```python
from build123d import *

# Parameters (mm, degrees)
SKETCH1_W                    = 120
SKETCH1_H                    = 72
BOSS_EXTRUDE1_DEPTH          = 10
FILLET1_R                    = 10
M12_TAPPED_HOLE1_D           = 10.2
M12_TAPPED_HOLE1_CSINK_D     = 12.05
M12_TAPPED_HOLE1_CSINK_ANGLE = 90
BOSS_EXTRUDE2_START          = 10
SKETCH4_W                    = 50
SKETCH4_H                    = 72
BOSS_EXTRUDE2_DEPTH          = 3
CUT_EXTRUDE1_DEPTH           = 72.168813395
CUT_EXTRUDE1_DEPTH_BACK      = 72.168813395


with BuildPart() as part:
    # Sketch1 → Boss-Extrude1 (new body)
    with BuildSketch(Plane(origin=(0, 0, 0), x_dir=(1, 0, 0), z_dir=(0, 1, 0))):
        Rectangle(SKETCH1_W, SKETCH1_H)
    extrude(amount=BOSS_EXTRUDE1_DEPTH)

    # Fillet1
    fillet1_edges = [part.edges().sort_by_distance(p)[0] for p in [
        (60, 5, 36),
        (-60, 5, 36),
        (-60, 5, -36),
        (60, 5, -36),
    ]]
    fillet(fillet1_edges, radius=FILLET1_R)

    # M12 Tapped Hole1 (through all)
    with Locations(Plane.XZ):
        with Locations((-50, -26), (50, -26), (50, 26), (-50, 26)):
            CounterSinkHole(M12_TAPPED_HOLE1_D / 2, M12_TAPPED_HOLE1_CSINK_D / 2, counter_sink_angle=M12_TAPPED_HOLE1_CSINK_ANGLE)

    # Sketch4 → Boss-Extrude2 (add)
    with BuildSketch(Plane(origin=(0, 0, 0), x_dir=(1, 0, 0), z_dir=(0, 1, 0)).offset(BOSS_EXTRUDE2_START)):
        Rectangle(SKETCH4_W, SKETCH4_H)
    extrude(amount=BOSS_EXTRUDE2_DEPTH)

    # Sketch5 → Cut-Extrude1 (cut, two sides: drawn at the far end of the back side and taken through both)
    with BuildSketch(Plane.XY.offset(-CUT_EXTRUDE1_DEPTH_BACK)):
        Polygon((-28, 0), (-25, 3), (25, 3), (28, 0), align=None)
    extrude(amount=CUT_EXTRUDE1_DEPTH + CUT_EXTRUDE1_DEPTH_BACK, mode=Mode.SUBTRACT)


solid = part.part
```
The listing builds one solid part. Answer for the finished solid, in the listing's coordinates (mm). A direction names the side the tool comes from. Coordinates: 2 decimals unless noted, no trailing zeros. Loops run counter-clockwise (first coordinate to the right, second up) from the corner with the lowest first, then second, coordinate; pieces in that order, holes last. Notation, with made-up numbers: M 46.25,79.25 L 66.25,79.25 A24 ccw 66.25,103.25 Z; hole C -17,7.5 d7. An arc over 180 degrees is marked long. Answer as a JSON object with one key per item and string values. Group by question number.
Item 1: Determine the mould class of faces 1 (the face through (0, 13, -1)), 2 (the face through (-27, 1, -1)), 3 (the face through (-57.15, 5.07, 32.99)) for opening direction X: +X half, -X half, draft (parallel to the pull), parting line (faces both ways), or undercut.
Item 2: Consider L1, parallel to X at y = 5.25, z = 26; L2, parallel to Z at x = 50, y = 4.75; L3, parallel to X at y = 6, z = -28.5. Determine where each line is inside the solid, lowest interval first.
Item 3: Which of the six approach directions +Z, -Z, +X, -X, +Y, -Y give full straight-line access (tool end or side, diameter ignored) to faces 4 (the face through (-25, 11, 1)), 5 (the face through (42, 10, -1)), 6 (the face through (26, 2, -1)), 7 (the face through (54.05, 5.53, -29.1))?
Item 4: Section B-B (x = 17.5) is taken. Write down the section's boundary in (y, z), and give its area (3 significant figures).
Item 5: Section C-C (y = 11.5) is taken. Write down the section's boundary in (x, z), and give its area (3 significant figures).
Item 6: Each of these flat-tipped pins is pushed along its axis until it touches: P1, Ø6, axis at x = -50, z = 26, coming from the -Y side (3 decimals); P2, Ø11.5, axis at x = -50, z = -26, coming from the +Y side; P3, Ø3, axis at x = -37, y = 10.5, coming from the +Z side; P4, Ø2, axis at x = 6.5, z = 25.5, coming from the -Y side. Where does it stop, or does it pass through?
Item 7: Section A-A (z = 4.5) is taken. Write down the section's boundary in (x, y), and give its area (3 significant figures).
Solved:
{
 "1": {"face 1": "draft", "face 2": "undercut", "face 3": "-X half"},
 "2": {"L1": "x = -60 to -55.1, -44.9 to 44.9, 55.1 to 60", "L2": "z = -36 to -31.1, -20.9 to 20.9, 31.1 to 36", "L3": "x = -59.68 to -54.45, -45.55 to 45.55, 54.45 to 59.68"},
 "3": {"face 4": "+Z, -Z, -X, +Y", "face 5": "+Z, -Z, +X, +Y", "face 6": "+Z, -Z, -Y", "face 7": "+Y, -Y"},
 "4": {"outline": "M 3,-36 L 13,-36 L 13,36 L 3,36 Z", "area": "720 mm2"},
 "5": {"outline": "M -25,-36 L 25,-36 L 25,36 L -25,36 Z", "area": "3,600 mm2"},
 "6": {"P1": "passes through", "P2": "stops at y = 10", "P3": "stops at z = 36", "P4": "stops at y = 3"},
 "7": {"outline": "M -60,0 L -28,0 L -25,3 L 25,3 L 28,0 L 60,0 L 60,10 L 25,10 L 25,13 L -25,13 L -25,10 L -60,10 Z", "area": "1,190 mm2"}
}
